```python
from build123d import *

# Parameters (mm, degrees)
F0_R     = 3
F1_DEPTH = 16
F3_DEPTH = 14
F4_W     = 20
F4_H     = 4
F5_DEPTH = 4
F6_R     = 3
F7_DEPTH = 25
F8_R     = 4
F9_DEPTH = 25


with BuildPart() as f1:
    # F0 (on Front) → F1 (new body, symmetric)
    with BuildSketch(Plane.XZ):
        with BuildLine():
            Line((-11.5073820825, 4), (-11.5073820825, 0))
            Line((-11.5073820825, 0), (39.4926179175, 0))
            Line((39.4926179175, 0), (39.4926179175, 11))
            ThreePointArc((39.4926179175, 11), (37.4423653858, 15.9497474683), (32.4926179175, 18))
            Line((32.4926179175, 18), (-6.5073820825, 18))
            Line((-6.5073820825, 18), (-6.5073820825, 14))
            Line((-6.5073820825, 14), (4.4926179175, 14))
            Line((4.4926179175, 14), (4.4926179175, 4))
            Line((4.4926179175, 4), (-11.5073820825, 4))
        make_face()
        with Locations((32.4926179175, 11)):
            Circle(F0_R, mode=Mode.SUBTRACT)
    extrude(amount=F1_DEPTH, both=True)

    # F2 (on face) → F3 (cut)
    with BuildSketch(Plane.XY.offset(18)):
        with BuildLine():
            Line((44.1028997302, 10), (32.4926179175, 10))
            Line((32.4926179175, 10), (17.4926179175, 10))
            ThreePointArc((17.4926179175, 10), (7.4926179175, 0), (17.4926179175, -10))
            Line((17.4926179175, -10), (32.4926179175, -10))
            Line((32.4926179175, -10), (44.1028997302, -10))
            Line((44.1028997302, -10), (44.1028997302, 10))
        make_face()
        with BuildLine():
            ThreePointArc((-6.5073820825, -10), (3.4926179175, 0), (-6.5073820825, 10))
            Line((-6.5073820825, 10), (-6.5073820825, -10))
        make_face()
    extrude(amount=-F3_DEPTH, mode=Mode.SUBTRACT)

    # F4 (on face) → F5 (cut)
    with BuildSketch(Plane.YZ.offset(39.4926179175)):
        with Locations((0, 2)):
            Rectangle(F4_W, F4_H)
    extrude(amount=-F5_DEPTH, mode=Mode.SUBTRACT)

    # F6 (on face) → F7 (cut)
    with BuildSketch(Plane.XY.offset(4)):
        with Locations((-5.5073820825, 0)):
            Circle(F6_R)
    extrude(amount=-F7_DEPTH, mode=Mode.SUBTRACT)

    # F8 (on face) → F9 (cut)
    with BuildSketch(Plane.XY.offset(4)):
        with Locations((17.4926179175, 0)):
            Circle(F8_R)
    extrude(amount=-F9_DEPTH, mode=Mode.SUBTRACT)


solid = f1.part
```
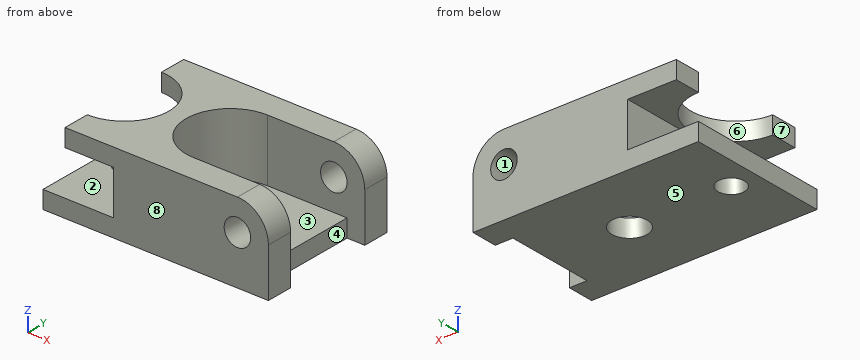
Design review of the part built by this model. Coordinates are the model's own, in mm. Face numbers are marked on the shaded views. A direction names the side the tool comes from. Give positions to 0.01 mm unless a question says otherwise; leave off trailing zeros. Order: outer loops, then holes, each group sorted by start corner. A loop starts at its lowest first (then second) coordinate and runs counter-clockwise, first axis right, second up. Notation, with made-up numbers: M 4,37.25 L 61,37.25 A9 ccw 61,43.25 Z; hole C 78.25,-28.5 d11. An arc over 180 degrees is marked long. One line per question, with ' | ' between items. Start each with the question number.
Q1. The part is to be moulded in two halves that separate along Y. For the marked faces 6, 7 and 8, say which applies: +Y half, -Y half, draft (parallel to the pull), parting line (faces both ways), or undercut.
Q2. We need section B-B (z = 9.5). Write out the cut boundary in (x, y).
Q3. We need section A-A (y = 0). Write out the cut boundary in (x, z).
Q4. For pin 1 Ø1 at (y, z) = (3.5, 15) entering from +X; pin 2 Ø2 at (y, z) = (13, 16.5) entering from -X; pin 3 Ø6 at (x, y) = (20.5, 0) entering from +Z; pin 4 Ø5 at (x, y) = (17.49, 0) entering from -Z, all flat-tipped, find the tip position at first contact; note any pin that passes through.
Q5. For L1, parallel to Z at x = -2, y = 14; L2, parallel to X at y = -13.85, z = 11; L3, parallel to Y at x = 37.5, z = 7.75, list the stretches that pass through material, from the lowest coordinate up. Write a range as [from, to].
Q6. We need section D-D (x = 8). Write out the cut boundary in (y, z), plus the area to 3 significant figures.
Q7. Machinability: for the marked faces 1, 2, 3, 4 and 5, which of the approach directions +Z, -Z, +X, -X, +Y, -Y give a long, thin tool a straight path to every point of the face, cutting with its end or side? Answer none if there is none.
Q8. We need section C-C (z = 4.75). Write out the cut boundary in (x, y), plus the area to 3 significant figures.
Returned:
1) face 6: undercut | face 7: draft | face 8: -Y half
2) outline: M 4.49,-16 L 29.89,-16 L 29.89,-10 L 17.49,-10 A10 cw 17.49,10 L 29.89,10 L 29.89,16 L 4.49,16 Z; M 35.09,-16 L 39.49,-16 L 39.49,-10 L 35.09,-10 Z; M 35.09,10 L 39.49,10 L 39.49,16 L 35.09,16 Z
3) outline: M -11.51,0 L -8.51,0 L -8.51,4 L -11.51,4 Z; M -2.51,0 L 13.49,0 L 13.49,4 L 7.49,4 L 7.49,18 L 3.49,18 L 3.49,14 L 4.49,14 L 4.49,4 L -2.51,4 Z; M 21.49,0 L 35.49,0 L 35.49,4 L 21.49,4 Z
4) pin 1: x = 8.33 | pin 2: x = -6.51 | pin 3: z = 4 | pin 4: through
5) L1: [0, 4], [14, 18] | L2: [4.49, 29.49], [35.49, 39.49] | L3: [-16, -10], [10, 16]
6) outline: M -16,0 L 16,0 L 16,18 L 3.14,18 L 3.14,4 L -3.14,4 L -3.14,18 L -16,18 Z | area: 488 mm2
7) face 1: +Y, -Y | face 2: -X, +Y, -Y | face 3: +Z, +X | face 4: +Z, -Z, +X | face 5: -Z, +X, -X, +Y, -Y
8) outline: M 4.49,-16 L 39.49,-16 L 39.49,-10 L 17.49,-10 A10 cw 17.49,10 L 39.49,10 L 39.49,16 L 4.49,16 Z | area: 523 mm2
